Build history of the part. All positions in model axes, mm. A direction names the side the tool comes from. Give positions to 0.01 mm unless a question says otherwise; leave off trailing zeros. Loops run counter-clockwise (first coordinate to the right, second up) from the corner with the lowest first, then second, coordinate; pieces in that order, holes last. Notation, with made-up numbers: M 20.25,-32.5 L 78.25,-32.5 A24 ccw 78.25,-20.5 Z; hole C -5,-17 d5. An arc over 180 degrees is marked long. Answer as a JSON object with one key per item and string values. Group by question number.
1. 3-axis set-ups, long thin cutter, end or side, ignore diameter. For faces 1 (the face through (12, -4.9, 0)), 2 (the face through (11, 17.5, 0)), 3 (the face through (32.5, 7, 27)): which of +Z, -Z, +X, -X, +Y, -Y reach the whole face in a straight line?
2. Slice it at A-A (z = 20.5). List the corners of the cut face in (x, y).
3. Slice it at C-C (z = 11.5). List the corners of the cut face in (x, y).
4. Mould opens along Y. For faces 4 (the face through (-24.9, 6, 35)), 5 (the face through (-1.5, 6, 11)), 6 (the face through (11, 37.5, 35)), 7 (the face through (40.115, -19.149, 35.465)) say: released by +Y, released by -Y, zero draft, split by the parting line, or undercut.
5. Drill centre lines: line 1 along Y through (x, z) = (42.5, 34.3); line 2 along X through (y, z) = (6, 36); line 3 along Y through (x, z) = (11.5, 10.5). Where is each one in solid material? Low to high. Write a range as [from, to].
6. Drop flat-ended pins along their axis: pin 1 Ø12 at (y, z) = (10.5, 3) entering from +X; pin 2 Ø10.5 at (x, z) = (2, 30) entering from -Y; pin 3 Ø11 at (x, z) = (6, 2.5) entering from +Y; pin 4 Ø1.5 at (y, z) = (7, -2.5) entering from -X. Give the stop position or say it passes through.
7. Slice it at B-B (x = -19.9). List the corners of the cut face in (y, z).
8. Slice it at D-D (x = -12.5). List the corners of the cut face in (y, z).
Autodesk Inventor part; units mm, degrees
ref_plane "Work Plane1" through (0, 0, 12) normal (0, 0, 1) x (1, 0, 0)
ref_plane "YZ Plane" through (0, 0, 0) normal (1, 0, 0) x (0, 1, 0)
ref_plane "XZ Plane" through (0, 0, 0) normal (0, 1, 0) x (-1, 0, 0)
sketch "Sketch1" plane through (0, 0, 0) normal (0, 0, 1) x (1, 0, 0)
  line L0 (0, 0) -> (22.6, 0)
  line L1 (22.6, 0) -> (22.6, 12.6)
  line L2 (22.6, 12.6) -> (0, 12.6)
  line L3 (0, 12.6) -> (0, 0)
  line L4 (-4.9, 17.5) -> (27.5, 17.5)
  line L5 (27.5, 17.5) -> (27.5, -4.9)
  line L6 (27.5, -4.9) -> (-4.9, -4.9)
  line L7 (-4.9, -4.9) -> (-4.9, 17.5)
  dimension "d0" = 22.6
  dimension "d1" = 12.6
  dimension "d2" = 4.9
extrude "Extrusion1" add sketch "Sketch1" along normal blind 17
sketch "Sketch2" plane through (0, 0, 0) normal (0, 0, -1) x (-1, 0, 0)
  line L0 (4.9, -4.9) -> (-27.5, -4.9)
  line L1 (-27.5, -4.9) -> (-27.5, 17.5)
  line L2 (-27.5, 17.5) -> (4.9, 17.5)
  line L3 (4.9, 17.5) -> (4.9, -4.9)
  point P0 (0, 0)
extrude "Extrusion2" add sketch "Sketch2" along normal blind 5
sketch "Sketch3" plane through (0, 0, 17) normal (0, 0, 1) x (1, 0, 0)
  line L0 (-4.9, -4.9) -> (27.5, -4.9)
  line L1 (27.5, -4.9) -> (27.5, 17.5)
  line L2 (27.5, 17.5) -> (-4.9, 17.5)
  line L3 (-4.9, 17.5) -> (-4.9, -4.9)
  line L4 (0, 0) -> (0, 12.6)
  line L5 (0, 12.6) -> (22.6, 12.6)
  line L6 (22.6, 12.6) -> (22.6, 0)
  line L7 (22.6, 0) -> (0, 0)
  line L8 (-9.9, -9.9) -> (32.5, -9.9)
  line L9 (32.5, -9.9) -> (32.5, 22.5)
  line L10 (32.5, 22.5) -> (-9.9, 22.5)
  line L11 (-9.9, 22.5) -> (-9.9, -9.9)
  line L12 (-4.9, 6.3) -> (-2.6, 6.3) construction
  line L13 (27.5, 17.5) -> (27.5, -4.9)
  line L14 (27.5, 6.3) -> (25.2, 6.3) construction
  circle A0 centre (-2.6, 6.3) radius 1
  circle A1 centre (25.2, 6.3) radius 1
  dimension "d7" = 5
  dimension "d10" = 2.3
  dimension "d11" = 2.3
  dimension "d12" = 2
  dimension "d13" = 2
extrude "Extrusion4" add sketch "Sketch3" along normal blind 5 contours A0 | A1
chamfer "Chamfer1" distance 0.5 angle 45 2 edges at (-3.6, 6.3, 22) (24.2, 6.3, 22)
ref_plane "Work Plane1" through (0, 0, 12) normal (0, 0, 1) x (1, 0, 0)
sketch "Sketch5" plane through (0, 0, 12) normal (0, 0, 1) x (1, 0, 0)
  line L0 (-4.9, -4.9) -> (27.5, -4.9)
  line L1 (27.5, -4.9) -> (27.5, 17.5)
  line L2 (27.5, 17.5) -> (-4.9, 17.5)
  line L3 (-4.9, 17.5) -> (-4.9, -4.9)
  line L4 (32.5, -9.9) -> (-9.9, -9.9)
  line L5 (-9.9, -9.9) -> (-9.9, 22.5)
  line L6 (-9.9, 22.5) -> (32.5, 22.5)
  line L7 (32.5, 22.5) -> (32.5, -9.9)
  point P0 (0, 0)
  dimension "d21" = 5
extrude "Extrusion5" add sketch "Sketch5" along normal blind 5
sketch "Sketch14" plane through (0, 0, 17) normal (0, 0, 1) x (1, 0, 0)
  line L0 (22.6, 12.6) -> (22.6, 0)
  line L1 (0, 12.6) -> (22.6, 12.6)
  line L2 (0, 0) -> (0, 12.6)
  line L3 (22.6, 0) -> (0, 0)
  line L4 (-9.9, -9.9) -> (-9.9, 22.5)
  line L5 (-9.9, 22.5) -> (32.5, 22.5)
  line L6 (32.5, 22.5) -> (32.5, -9.9)
  line L7 (32.5, -9.9) -> (-9.9, -9.9)
  line L8 (-14.9, -14.9) -> (-14.9, 27.5)
  line L9 (-14.9, 27.5) -> (37.5, 27.5)
  line L10 (37.5, 27.5) -> (37.5, -14.9)
  line L11 (37.5, -14.9) -> (-14.9, -14.9)
  dimension "d52" = 9.9
  dimension "d53" = 5
extrude "Extrusion11" add sketch "Sketch14" along normal blind 16 contours L8 L9 L10 L11
sketch "Sketch15" plane through (0, 0, 33) normal (0, 0, 1) x (1, 0, 0)
  line L0 (-14.9, 27.5) -> (-14.9, -14.9)
  line L1 (-14.9, -14.9) -> (37.5, -14.9)
  line L2 (37.5, -14.9) -> (37.5, 27.5)
  line L3 (37.5, 27.5) -> (-14.9, 27.5)
  line L4 (47.5, -24.9) -> (-24.9, -24.9)
  line L5 (-24.9, -24.9) -> (-24.9, 37.5)
  line L6 (-24.9, 37.5) -> (47.5, 37.5)
  line L7 (47.5, 37.5) -> (47.5, -24.9)
  line L8 (32.5, -9.9) -> (-9.9, -9.9)
  line L9 (-9.9, -9.9) -> (-9.9, 22.5)
  line L10 (-9.9, 22.5) -> (32.5, 22.5)
  line L11 (32.5, 22.5) -> (32.5, -9.9)
  point P0 (0, 0)
  dimension "d56" = 10
extrude "Extrusion12" add sketch "Sketch15" along normal blind 5 contours L3 L2 L1 L0 | L4 L5 L6 L7
sketch "Sketch16" plane through (0, 0, 33) normal (0, 0, -1) x (-1, 0, 0)
  line L0 (-37.5, -14.9) -> (-37.5, 27.5)
  line L1 (14.9, -14.9) -> (-37.5, -14.9)
  line L2 (14.9, 27.5) -> (14.9, -14.9)
  line L3 (-37.5, 27.5) -> (14.9, 27.5)
  line L4 (9.9, 22.5) -> (9.9, -9.9)
  line L5 (9.9, -9.9) -> (-32.5, -9.9)
  line L6 (-32.5, -9.9) -> (-32.5, 22.5)
  line L7 (-32.5, 22.5) -> (9.9, 22.5)
  line L8 (-42.5, 32.5) -> (-42.5, -19.9) construction
  line L9 (-42.5, -19.9) -> (19.9, -19.9) construction
  line L10 (19.9, -19.9) -> (19.9, 32.5) construction
  line L11 (19.9, 32.5) -> (-42.5, 32.5) construction
  circle A0 centre (19.9, 6.3) radius 2.5
  circle A1 centre (-42.5, 32.5) radius 2.5
  circle A2 centre (-42.5, -19.9) radius 2.5
  point P0 (0, 0)
  dimension "d59" = 5
  dimension "d60" = 5
  dimension "d61" = 5
  dimension "d62" = 5
extrude "Extrusion13" cut sketch "Sketch16" against normal blind 5 contours A0 | A1 | A2
sketch "Sketch17" plane through (-4.9, -4.9, -5) normal (-1, 0, 0) x (0, 0, 1)
  line L0 (-10, 15.2) -> (10, 15.2)
  line L1 (10, 15.2) -> (10, 7.2)
  line L2 (10, 7.2) -> (-10, 7.2)
  line L3 (-10, 7.2) -> (-10, 15.2)
  line L4 (0, 22.4) -> (0, 0)
  line L5 (-10, 15.2) -> (10, 7.2) construction
  line L6 (10, 15.2) -> (-10, 7.2) construction
  line L7 (5, 15.2) -> (5, 7.2)
  line L8 (0, 11.2) -> (5, 11.2)
  point P0 (5, 4.9)
  dimension "d65" = 20
  dimension "d66" = 8
  dimension "d67" = 5
extrude "Extrusion14" cut sketch "Sketch17" against normal blind 5 contours L0 L1 L2 L7
sketch "Sketch18" plane through (0, 0, 12) normal (0, 0, -1) x (-1, 0, 0)
  line L0 (-32.5, 22.5) -> (9.9, 22.5)
  line L1 (-32.5, -9.9) -> (-32.5, 22.5)
  line L2 (9.9, -9.9) -> (-32.5, -9.9)
  line L3 (9.9, 22.5) -> (9.9, -9.9)
  line L4 (4.9, -4.9) -> (4.9, 17.5)
  line L5 (-27.5, -4.9) -> (4.9, -4.9)
  line L6 (-27.5, 17.5) -> (-27.5, -4.9)
  line L7 (4.9, 17.5) -> (-27.5, 17.5)
  point P0 (0, 0)
extrude "Extrusion15" add sketch "Sketch18" along normal blind 7
sketch "Sketch20" plane through (-4.9, -4.9, -5) normal (-1, 0, 0) x (0, 0, 1)
  line L0 (5, 7.2) -> (0, 7.2)
  line L1 (5, 15.2) -> (10, 15.2)
  line L2 (5, 15.2) -> (0, 15.2)
  line L3 (0, 15.2) -> (0, 7.2)
  line L4 (5, 15.2) -> (5, 17.5)
  line L5 (5, 7.2) -> (5, 15.2)
  point P0 (5, 4.9)
  dimension "d74" = 10
extrude "Extrusion17" cut sketch "Sketch20" against normal blind 12
sketch "Sketch21" plane through (0, 0, 17) normal (0, 0, -1) x (-1, 0, 0)
  line L0 (-32.5, -9.9) -> (9.9, -9.9)
  line L1 (9.9, -9.9) -> (9.9, 22.5)
  line L2 (9.9, 22.5) -> (-32.5, 22.5)
  line L3 (-32.5, 22.5) -> (-32.5, -9.9)
  line L4 (0, 2.3) -> (0, 10.3)
  line L5 (4.9, 2.3) -> (0, 2.3)
  line L6 (4.9, -4.9) -> (4.9, 2.3)
  line L7 (-27.5, -4.9) -> (4.9, -4.9)
  line L8 (-27.5, 17.5) -> (-27.5, -4.9)
  line L9 (4.9, 17.5) -> (-27.5, 17.5)
  line L10 (4.9, 10.3) -> (4.9, 17.5)
  line L11 (4.9, 10.3) -> (0, 10.3)
  line L12 (-37.5, -14.9) -> (-37.5, 27.5)
  line L13 (14.9, -14.9) -> (-37.5, -14.9)
  line L14 (14.9, 27.5) -> (14.9, -14.9)
  line L15 (-37.5, 27.5) -> (14.9, 27.5)
  line L16 (9.9, 22.5) -> (9.9, -9.9)
  line L17 (9.9, -9.9) -> (-32.5, -9.9)
  line L18 (-32.5, -9.9) -> (-32.5, 22.5)
  line L19 (-32.5, 22.5) -> (9.9, 22.5)
  point P0 (0, 0)
extrude "Extrusion18" add sketch "Sketch21" along normal blind 12 contours L12 L15 L14 L13
sketch "Sketch22" plane through (0, 0, 17) normal (0, 0, 1) x (1, 0, 0)
  line L0 (0, 12.6) -> (22.6, 12.6)
  line L1 (22.6, 12.6) -> (22.6, 0)
  line L2 (22.6, 0) -> (0, 0)
  line L3 (0, 0) -> (0, 12.6)
  line L4 (24.1, 14.1) -> (-1.5, 14.1)
  line L5 (-1.5, 14.1) -> (-1.5, -1.5)
  line L6 (-1.5, -1.5) -> (24.1, -1.5)
  line L7 (24.1, -1.5) -> (24.1, 14.1)
  dimension "d79" = 1.5
extrude "Extrusion19" cut sketch "Sketch22" against normal blind 17
sketch "Sketch23" plane through (0, 0, 38) normal (0, 0, 1) x (1, 0, 0)
  circle A0 centre (-19.9, 6.3) radius 2.5
  circle A1 centre (42.5, 32.5) radius 2.5
  circle A2 centre (42.5, -19.9) radius 2.5
  line L0 (47.5, 37.5) -> (-24.9, 37.5)
  line L1 (-24.9, 37.5) -> (-24.9, -24.9)
  line L2 (-24.9, -24.9) -> (47.5, -24.9)
  line L3 (47.5, -24.9) -> (47.5, 37.5)
  line L4 (32.5, -9.9) -> (-9.9, -9.9)
  line L5 (-9.9, -9.9) -> (-9.9, 22.5)
  line L6 (-9.9, 22.5) -> (32.5, 22.5)
  line L7 (32.5, 22.5) -> (32.5, -9.9)
  point P0 (0, 0)
equation "\"d63\" = d62"
equation "\"d68\" = d62"
properties part number "servo_holder_V2_3DPrint"
Established:
{
 "1": {"face 1": "-Z, +X, -X, -Y", "face 2": "-Z, +X, -X, +Y", "face 3": "+Z"},
 "2": {"outline": "M -14.9,-14.9 L 37.5,-14.9 L 37.5,27.5 L -14.9,27.5 Z; C -2.6,6.3 d2; C 25.2,6.3 d2; hole M -9.9,-9.9 L 32.5,-9.9 L 32.5,22.5 L -9.9,22.5 Z"},
 "3": {"outline": "M -14.9,-14.9 L 37.5,-14.9 L 37.5,27.5 L -14.9,27.5 Z; hole M -1.5,-1.5 L 24.1,-1.5 L 24.1,14.1 L -1.5,14.1 Z"},
 "4": {"face 4": "zero draft", "face 5": "undercut", "face 6": "released by +Y", "face 7": "undercut"},
 "5": {"line 1": "y = [-24.9, -22.4], [-17.4, 30], [35, 37.5]", "line 2": "x = [-24.9, -22.38], [-17.42, -9.9], [32.5, 47.5]", "line 3": "y = [-14.9, -1.5], [14.1, 27.5]"},
 "6": {"pin 1": "stops at x = 37.5", "pin 2": "stops at y = -24.9", "pin 3": "stops at y = 27.5", "pin 4": "stops at x = 7.1"},
 "7": {"outline": "M -24.9,33 L 3.8,33 L 3.8,38 L -24.9,38 Z; M 8.8,33 L 37.5,33 L 37.5,38 L 8.8,38 Z"},
 "8": {"outline": "M -24.9,33 L -14.9,33 L -14.9,5 L 27.5,5 L 27.5,33 L 37.5,33 L 37.5,38 L -24.9,38 Z"}
}
